Check sheet for the modelled part. Datum: model origin and axes. Units: mm. A direction names the side the tool comes from. Give positions to 0.01 mm unless a question says otherwise; leave off trailing zeros. Loops run counter-clockwise (first coordinate to the right, second up) from the corner with the lowest first, then second, coordinate; pieces in that order, holes last. Notation, with made-up numbers: (55.25, 16.25) -> (73.25, 16.25) arc R7 ccw to (73.25, 28.25) -> close; hole circle Ø3 at (-11, -35.75). An arc over 180 degrees is marked (long way). Write each question's results on one line, items separated by ' | '. Start each with the question number.
1. Cross-section at A-A on x = 44. Record the boundary of the cut face in (y, z), and give its area (3 significant figures).
2. Tool access check on faces 1 (the face through (55, 0, 10)), 2 (the face through (57.31, -0.96, 7.46)). Record the directions out of +Z, -Z, +X, -X, +Y, -Y that give a thin tool (end or side, any length) a straight path to the whole face; none if there is none.
3. Mould release check, pull along X, two halves, no side actions. Record for faces 3 (the face through (150, -1, 2)), 4 (the face through (-0.54, -2.44, 7.46)), 5 (the face through (-82.5, 0.1, 7.5)), 6 (the face through (-2, 50, 2)): +X half, -X half, draft (parallel to the pull), parting line (faces both ways), or undercut.
4. Gauge pin test, flat end, axial feed: pin 1 Ø5 at (x, y) = (54.5, 35.5) entering from +Z. Record the tip position at first contact, or that the pin passes through.
5. Material ranges on L1, parallel to X at y = 1.5, z = 5.75; L2, parallel to X at y = 1, z = 8.5; L3, parallel to Z at x = 44.5, y = -26, recorded low to high. Write a range as from..to.
6. Cross-section at B-B on y = -12.5. Record the boundary of the cut face in (x, z).
from build123d import *

# Parameters (mm, degrees)
F0_W     = 300
F0_H     = 100
F1_DEPTH = 5
F2_R     = 2.5
F3_DEPTH = 5
F4_DEPTH = 5


with BuildPart() as f1:
    # F0 (on Top) → F1 (new body)
    with BuildSketch(Plane.XY):
        Rectangle(F0_W, F0_H)
    extrude(amount=F1_DEPTH)

    # F2 (on face) → F3 (join)
    with BuildSketch(Plane.XY.offset(5)):
        Circle(F2_R)
        with Locations((-80, 0)):
            Circle(F2_R)
    extrude(amount=F3_DEPTH)

    # F2 (on face) → F4 (join)
    with BuildSketch(Plane.XY.offset(5)):
        Circle(F2_R)
        with Locations((-80, 0)):
            Circle(F2_R)
        with Locations((55, 0)):
            Circle(F2_R)
    extrude(amount=F4_DEPTH)


solid = f1.part
Geometry says:
1) outline: (-50, 0) -> (50, 0) -> (50, 5) -> (-50, 5) -> close | area: 500 mm^2
2) face 1: +Z, +X, -X, +Y, -Y | face 2: +Z
3) face 3: +X half | face 4: undercut | face 5: undercut | face 6: draft
4) pin 1: z = 5
5) L1: -82..-78, -2..2, 53..57 | L2: -82.29..-77.71, -2.29..2.29, 52.71..57.29 | L3: 0..5
6) outline: (-150, 0) -> (150, 0) -> (150, 5) -> (-150, 5) -> close
